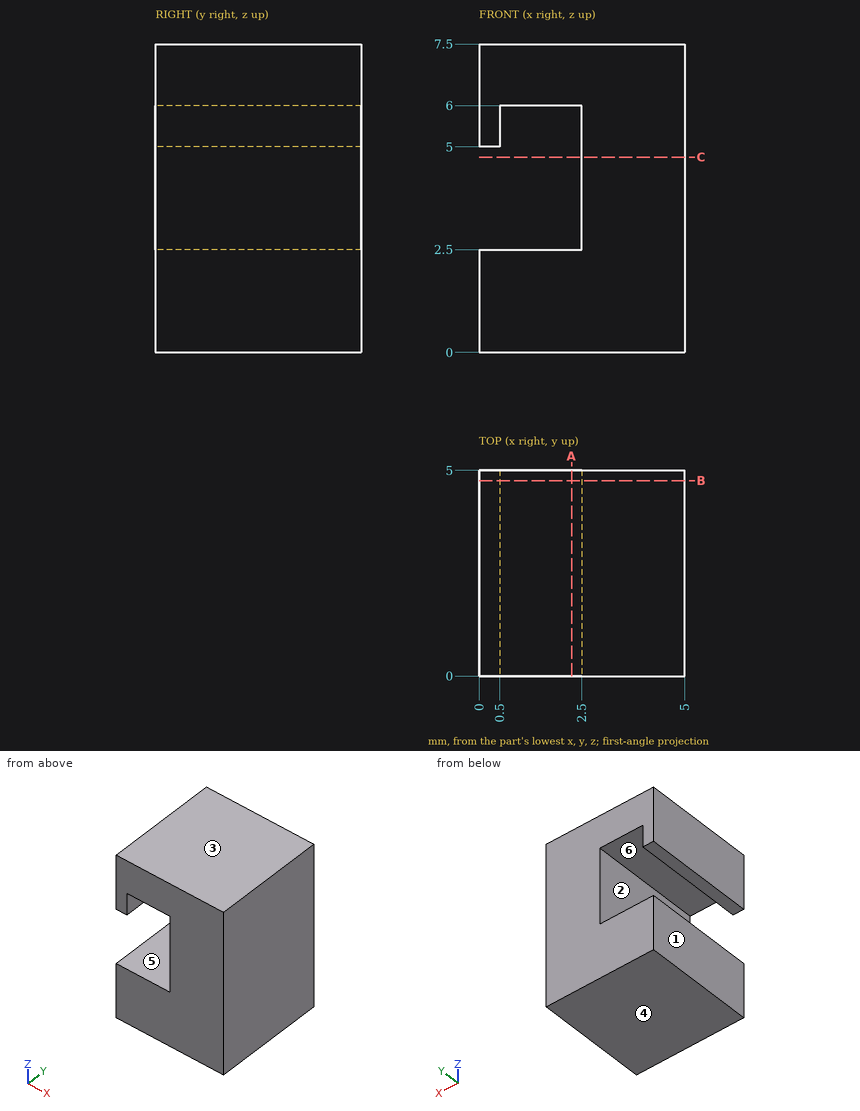
Part print with two shaded views. Sizes in mm from the minimum x, y, z corner. A direction names the side the tool comes from. Round coordinates to 2 decimals unless told otherwise and drop trailing zeros. Order: outer loops, then holes, each group sorted by start corner. A loop starts at its lowest first (then second) coordinate and runs counter-clockwise, first axis right, second up. Notation, with made-up numbers: M 71.5,-24.75 L 115.5,-24.75 A18 ccw 115.5,-5.75 Z; hole C 31.25,-28 d11. An arc over 180 degrees is marked long. Put each result on its own line as item: value. Start each with the question number.
1. Two-plate mould, pull along X, no slides. Class the marked faces 1, 2 and 3: +X half, -X half, draft (parallel to the pull), parting line (faces both ways), or undercut.
2. Slice it at C-C on z = 4.75. List the corners of the cut face in (x, y), then the cut area to 3 significant figures.
3. Tool access for the marked faces 4, 5 and 6: list every direction of +Z, -Z, +X, -X, +Y, -Y with a clear straight run to the whole face (end or side of a thin tool).
4. Slice it at B-B on y = 4.75. List the corners of the cut face in (x, z).
5. Drop a flat-ended pin along its axis: pin 1 (2 mm diameter, centred on x = 2.5, y = 2, fed in from -Z). Give the stop position or say it passes through.
6. Drill centre lines: probe 1 along X at (y, z) = (3.5, 5.5); probe 2 along Z at (x, y) = (1.9, 0.5); probe 3 along X at (y, z) = (1.85, 4). Where is each one in solid material? Low to high. Write a range as [from, to].
7. Slice it at A-A on x = 2.25. List the corners of the cut face in (y, z).
Findings:
1. face 1: -X half
1. face 2: undercut
1. face 3: draft
2. outline: M 2.5,0 L 5,0 L 5,5 L 2.5,5 Z
2. area: 12.5 mm2
3. face 4: -Z, +X, -X, +Y, -Y
3. face 5: -X, +Y, -Y
3. face 6: +Y, -Y
4. outline: M 0,0 L 5,0 L 5,7.5 L 0,7.5 L 0,5 L 0.5,5 L 0.5,6 L 2.5,6 L 2.5,2.5 L 0,2.5 Z
5. pin 1: z = 0
6. probe 1: [0, 0.5], [2.5, 5]
6. probe 2: [0, 2.5], [6, 7.5]
6. probe 3: [2.5, 5]
7. outline: M 0,0 L 5,0 L 5,2.5 L 0,2.5 Z; M 0,6 L 5,6 L 5,7.5 L 0,7.5 Z
